```python
from build123d import *

# Parameters (mm, degrees)
F1_W        = 42
F1_H        = 9
F2_DEPTH    = 7
F3_R        = 4.1
F4_DEPTH    = 25
F5_T1_DEPTH = 26.0282480506
F7_DEPTH    = 25
F8_W        = 10
F8_H        = 9
F9_DEPTH    = 15
F10_R       = 1.5
F11_DEPTH   = 25
F12_R       = 2


# Not quite as in the source:
# - a fillet or chamfer that OpenCascade refuses, or shapes differently, is made with other operations: its cross-section is extruded or revolved along the edge and cut away or added


with BuildPart() as f2:
    # F1 (on Top) → F2 (new body)
    with BuildSketch(Plane.XY):
        with Locations((21, 4.5)):
            Rectangle(F1_W, F1_H)
    extrude(amount=F2_DEPTH)

    # F3 (on face) → F4 (cut)
    with BuildSketch(Plane.XY.offset(7)):
        with Locations((15, 3.6)):
            Circle(F3_R)
    extrude(amount=-F4_DEPTH, mode=Mode.SUBTRACT)

    # F5: chamfer of 7 on 2 edges, made by hand

    # F5_s2 → F5_t1 (cut)
    with BuildSketch(Plane.XY.offset(-9.5141240253)):
        with BuildLine():
            Line((20.7610452751, -0.2264961011), (18.73515334, 2.5608842714))
            Line((18.73515334, 2.5608842714), (18.6019903715, 2.6041002851))
            ThreePointArc((18.6019903715, 2.6041002851), (18.0707550937, 1.0995874031), (16.895141727, 0.1229268293))
            Line((16.895141727, 0.1229268293), (16.962141687, -0.14))
            ThreePointArc((16.962141687, -0.14), (18.861593481, -0.14), (20.7610452751, -0.3664961011))
            Line((20.7610452751, -0.3664961011), (20.7610452751, -0.2264961011))
        make_face()
        with BuildLine():
            Line((11.26484666, 2.5608842714), (9.2389547249, -0.2264961011))
            Line((9.2389547249, -0.2264961011), (9.2389547249, -0.3664961011))
            ThreePointArc((9.2389547249, -0.3664961011), (11.138406519, -0.14), (13.037858313, -0.14))
            Line((13.037858313, -0.14), (13.104858273, 0.1229268293))
            ThreePointArc((13.104858273, 0.1229268293), (11.9292449063, 1.0995874031), (11.3980096285, 2.6041002851))
            Line((11.3980096285, 2.6041002851), (11.26484666, 2.5608842714))
        make_face()
    extrude(amount=F5_T1_DEPTH, mode=Mode.SUBTRACT)

    # F6 (on face) → F7 (cut)
    with BuildSketch(Plane(origin=(0, 9, 0), x_dir=(-1, 0, 0), z_dir=(0, 1, 0))):
        with BuildLine():
            Line((-5.5, 3.5), (-3.825, 3.5))
            ThreePointArc((-3.825, 3.5), (-4.3155961415, 4.6844038585), (-5.5, 5.175))
            Line((-5.5, 5.175), (-5.5, 3.5))
        make_face()
        with BuildLine():
            ThreePointArc((-5.5, 1.825), (-4.3155961415, 2.3155961415), (-3.825, 3.5))
            Line((-3.825, 3.5), (-5.5, 3.5))
            Line((-5.5, 3.5), (-5.5, 1.825))
        make_face()
        with BuildLine():
            Line((-5.5, 3.5), (-5.5, 5.175))
            ThreePointArc((-5.5, 5.175), (-7.175, 3.5), (-5.5, 1.825))
            Line((-5.5, 1.825), (-5.5, 3.5))
        make_face()
        with BuildLine():
            ThreePointArc((-38.175, 3.5), (-36.5, 1.825), (-34.825, 3.5))
            ThreePointArc((-34.825, 3.5), (-36.5, 5.175), (-38.175, 3.5))
        make_face()
    extrude(amount=-F7_DEPTH, mode=Mode.SUBTRACT)

    # F8 (on face) → F9 (join)
    with BuildSketch(Plane.XY.offset(7)):
        with Locations((37, 4.5)):
            Rectangle(F8_W, F8_H)
    extrude(amount=F9_DEPTH)

    # F10 (on face) → F11 (cut)
    with BuildSketch(Plane.YZ.offset(42)):
        with Locations((4.5, 19.5)):
            Circle(F10_R)
    extrude(amount=-F11_DEPTH, mode=Mode.SUBTRACT)

    # F12
    f12_edges = [f2.edges().sort_by_distance(p)[0] for p in [
        (37, 0, 22),
        (37, 9, 22),
    ]]
    fillet(f12_edges, radius=F12_R)


solid = f2.part
```
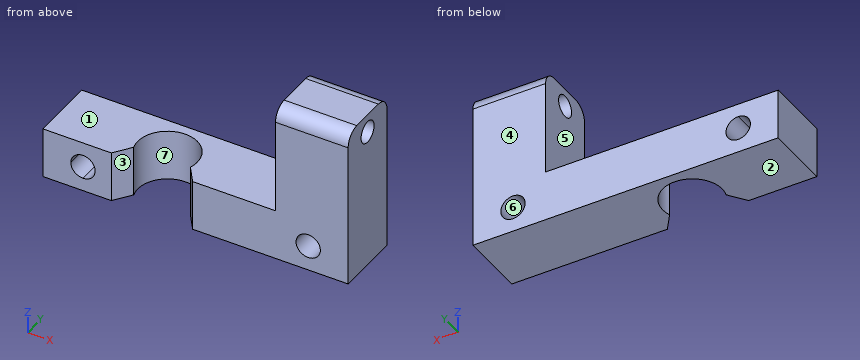
Part model, mm, in its own coordinate system. Face numbers are marked on the shaded views. A direction names the side the tool comes from. Round coordinates to 2 decimals unless told otherwise and drop trailing zeros. Write each loop counter-clockwise with the first axis right and the second up, starting at its lowest first coordinate (ties: lowest second). Pieces come first, ordered by that corner, then holes. Notation, with made-up numbers: (64, 63) -> (104, 63) arc R25 ccw to (104, 99) -> close; hole circle Ø2 at (32.25, -36). An arc over 180 degrees is marked (long way). Return JSON: item names as keys, results as strings. Group by question number.
Q1. Saw through at B-B on x = 36.5. Write the cut outline in (y, z) (3 decimals).
Q2. Probe L1, parallel to Z at x = 36.5, y = 2 (3 decimals); L2, parallel to Z at x = 37.75, y = 4.5; L3, parallel to Z at x = 37.25, y = 4.5. List the from-to ranges inside material, lowest first. Write a range as [from, to].
Q3. Mould opens along X. For the marked faces 4, 5, 6 and 7 say: pulls with the +X half, pulls with the -X half, needs draft (parallel to the pull), parting line crosses it, or undercut.
Q4. Saw through at D-D on y = 1.25. Write the cut outline in (x, z) (3 decimals).
Q5. Which spindle directions (+Z, -Z, +X, -X, +Y, -Y) get a long thin tool onto all of the face, cutting with end or side? Do the marked faces 1, 2 and 3. Say none if no direction does.
Q6. Pin check, flat tip, straight feed: pin 1 (2.5 mm diameter, centred on x = 24, y = 2.5, fed in from +Z). Stop position of the tip, or through.
Q7. Saw through at C-C on z = 19.5. Write the cut outline in (x, y), plus the area to 3 significant figures.
Q8. Saw through at A-A on y = 4.5. Write the cut outline in (x, z) (3 decimals).
Answer:
{
 "1": {"outline": "(0, 0) -> (9, 0) -> (9, 1.825) -> (0, 1.825) -> close; (0, 5.175) -> (9, 5.175) -> (9, 20) arc R2 ccw to (7, 22) -> (2, 22) arc R2 ccw to (0, 20) -> close; hole circle Ø3 at (4.5, 19.5)"},
 "2": {"L1": "[0, 1.825], [5.175, 22]", "L2": "[0, 2.39], [4.61, 18], [21, 22]", "L3": "[0, 2], [5, 18], [21, 22]"},
 "3": {"face 4": "needs draft", "face 5": "pulls with the -X half", "face 6": "undercut", "face 7": "undercut"},
 "4": {"outline": "(0, 0) -> (10.312, 0) -> (10.312, 7) -> (0, 7) -> close; (19.688, 0) -> (42, 0) -> (42, 21.854) -> (32, 21.854) -> (32, 7) -> (19.688, 7) -> close; hole circle Ø3.35 at (5.5, 3.5); hole circle Ø3.35 at (36.5, 3.5)"},
 "5": {"face 1": "+Z, -X, +Y, -Y", "face 2": "-Z, +X, -X, +Y, -Y", "face 3": "+Z, -Z, -Y"},
 "6": {"pin 1": "z = 7"},
 "7": {"outline": "(32, 0) -> (42, 0) -> (42, 3) -> (32, 3) -> close; (32, 6) -> (42, 6) -> (42, 9) -> (32, 9) -> close", "area": "60.0 mm2"},
 "8": {"outline": "(0, 0) -> (11, 0) -> (11, 7) -> (0, 7) -> close; (19, 0) -> (42, 0) -> (42, 18) -> (32, 18) -> (32, 7) -> (19, 7) -> close; (32, 21) -> (42, 21) -> (42, 22) -> (32, 22) -> close; hole circle Ø3.35 at (5.5, 3.5); hole circle Ø3.35 at (36.5, 3.5)"}
}
